Can you work these out from the model? Positions are in its coordinate system, mm. Coordinates: 2 decimals unless noted, no trailing zeros. Loops run counter-clockwise (first coordinate to the right, second up) from the corner with the lowest first, then second, coordinate; pieces in that order, holes last. Notation, with made-up numbers: (-3.75, 28.25) -> (16.25, 28.25) arc R16 ccw to (16.25, 57.25) -> close; hole circle Ø7 at (-2, 86). An arc over 180 degrees is marked (long way). Put each result on its own line as item: value. Start each with the question number.
Item 1: If we section it at A-A on x = 0: Please give me the cut outline in (y, z).
Item 2: If we section it at B-B on z = 12: Please give me the cut outline in (x, y), plus the area to 3 significant figures.
Item 3: We'd pull the mould along Y, two halves only. Please class faces 1 (the flat face through (-2, 2, 22.86)), 2 (the cylindrical face through (125.829, 39.626, 10.018)), 3 (the flat face through (-2, 2, 25.4)), 4 (the cylindrical face through (123.407, 38.863, 11.27)): pulls with the +Y half, pulls with the -Y half, needs draft (parallel to the pull), parting line crosses it, or undercut.
Item 4: Please list where these lines run through material, in increasing order: L1, parallel to Y at x = 0, z = 12.5; L2, parallel to Y at x = -80, z = 11.5; L3, parallel to X at y = 67, z = 20.5. Write a range as from..to.
Item 5: Will these pins go through, and if not, where does the flat tip stop? P1, Ø5, axis at y = -52, z = 22, coming from the -X side; P2, Ø5, axis at x = -19, z = 16.5, coming from the -Y side; P3, Ø6, axis at y = -83.5, z = 17, coming from the -X side.
```python
from build123d import *

# Parameters (mm, degrees)
F0_R     = 131.921172
F1_DEPTH = 25.4
F2_T     = -2.54
F3_R     = 5.08


with BuildPart() as f1:
    # F0 (on Top) → F1 (new body)
    with BuildSketch(Plane.XY):
        Circle(F0_R)
    extrude(amount=F1_DEPTH)

    # F2
    f2_openings = [f1.faces().sort_by_distance(p)[0] for p in [
        (0, 0, 0),
    ]]
    offset(amount=F2_T, openings=f2_openings)

    # F3
    f3_edges = [f1.edges().sort_by_distance(p)[0] for p in [
        (-131.921172, 0, 25.4),
    ]]
    fillet(f3_edges, radius=F3_R)


solid = f1.part
```
Solutions:
1. outline: (-131.92, 0) -> (-129.38, 0) -> (-129.38, 22.86) -> (129.38, 22.86) -> (129.38, 0) -> (131.92, 0) -> (131.92, 20.32) arc R5.08 ccw to (126.84, 25.4) -> (-126.84, 25.4) arc R5.08 ccw to (-131.92, 20.32) -> close
2. outline: circle Ø263.84 at (0, 0); hole circle Ø258.76 at (0, 0)
2. area: 2,090 mm^2
3. face 1: undercut
3. face 2: parting line crosses it
3. face 3: needs draft
3. face 4: undercut
4. L1: -131.92..-129.38, 129.38..131.92
4. L2: -104.9..-101.68, 101.68..104.9
4. L3: -113.64..-110.68, 110.68..113.64
5. P1: x = -122.15
5. P2: y = -130.89
5. P3: x = -104.51
